Geometry check sheet. Reference: drawing and pictorial views, mm from the part's lowest x, y, z. Coordinates: 2 decimals unless noted, no trailing zeros. Order: outer loops, then holes, each group sorted by start corner. A loop starts at its lowest first (then second) coordinate and runs counter-clockwise, first axis right, second up. Notation, with made-up numbers: M 12.5,14 L 68.5,14 A9 ccw 68.5,27 Z; hole C 14,48.25 d8. An arc over 180 degrees is marked long. Return JSON: item names as keys, results as strings.
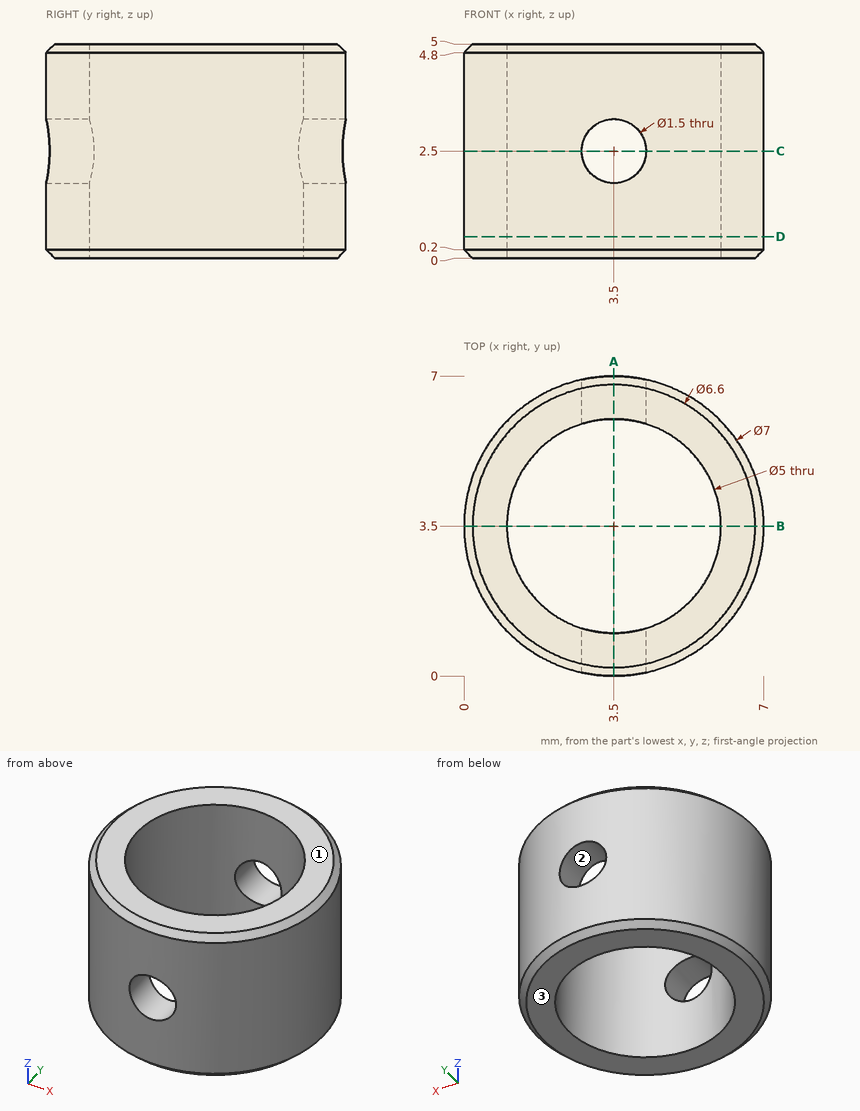
Q1. Draft check along Z on the marked faces 1, 2 and 3. Enter one of: pulls with the +Z half, pulls with the -Z half, needs draft (parallel to the pull), parting line crosses it, or undercut.
Values:
{"face 1": "pulls with the +Z half", "face 2": "undercut", "face 3": "pulls with the -Z half"}
Q2. Go/stop test with a flat-tipped pin: pin 1 (2 mm diameter, centred on x = 3.5, z = 2.5, fed in from -Y). Record where the tip stops, or that it passes through.
Values:
{"pin 1": "y = 0"}
Q3. Cross-section at D-D, the plane z = 0.5. Record the boundary of the cut face in (x, y), and give its area (3 significant figures).
Values:
{"outline": "C 3.5,3.5 d7; hole C 3.5,3.5 d5", "area": "18.8 mm^2"}
Q4. Cross-section at B-B, the plane y = 3.5. Record the boundary of the cut face in (x, z).
Values:
{"outline": "M 0,0.2 L 0.2,0 L 1,0 L 1,5 L 0.2,5 L 0,4.8 Z; M 6,0 L 6.8,0 L 7,0.2 L 7,4.8 L 6.8,5 L 6,5 Z"}
Q5. Cross-section at A-A, the plane x = 3.5. Record the boundary of the cut face in (y, z), and give its area (3 significant figures).
Values:
{"outline": "M 0,0.2 L 0.2,0 L 1,0 L 1,1.75 L 0,1.75 Z; M 0,3.25 L 1,3.25 L 1,5 L 0.2,5 L 0,4.8 Z; M 6,0 L 6.8,0 L 7,0.2 L 7,1.75 L 6,1.75 Z; M 6,3.25 L 7,3.25 L 7,4.8 L 6.8,5 L 6,5 Z", "area": "6.92 mm^2"}
Q6. Cross-section at C-C, the plane z = 2.5. Record the boundary of the cut face in (x, y).
Values:
{"outline": "M 2.75,0.08 L 2.75,1.12 A2.5 cw 2.75,5.88 L 2.75,6.92 A3.5 ccw Z; M 4.25,0.08 A3.5 ccw 4.25,6.92 L 4.25,5.88 A2.5 cw 4.25,1.12 Z"}
Q7. Material ranges on line 1 along Y through (x, z) = (3.5, 3.7); line 2 along X through (y, z) = (0.4, 2.5); line 3 along Y through (x, z) = (2.75, 4.25), recorded low to high.
Values:
{"line 1": "0 to 1, 6 to 7", "line 2": "1.88 to 2.75, 4.25 to 5.12", "line 3": "0.08 to 1.12, 5.88 to 6.92"}
